```python
from build123d import *

# Parameters (mm, degrees)
F0_W          = 3
F0_H          = 80
F2_R          = 12.5
F3_DEPTH      = 119.80777
F4_R          = 15
F5_DEPTH      = 102.88035
F4_R_2        = 18
F6_DEPTH      = 2
F6_DEPTH_BACK = 28
F7_R          = 1.99999


# Not quite as in the source:
# - a fillet or chamfer is up to 0.001 mm smaller than in the source, because OpenCascade refuses the exact size


with BuildPart() as f1:
    # F0 (on Front) → F1 (revolve)
    with BuildSketch(Plane.XZ):
        with Locations((11.5, -40)):
            Rectangle(F0_W, F0_H)
        with BuildLine():
            Line((10, -80), (10, 0))
            Line((10, 0), (0, 0))
            Line((0, 0), (-10, 0))
            Line((-10, 0), (-10, -80))
            add(Edge.make_bspline(
                [(-10, -80), (-6, -75.3330111863), (0, -64.6669888505), (6, -75.3330111128), (10, -80)],
                knots=[0, 0, 0, 0, 0.5, 1, 1, 1, 1], degree=3))
        make_face()
        with Locations((-11.5, -40)):
            Rectangle(F0_W, F0_H)
    revolve(axis=Axis((-1.5, 0, 0), (-1, 0, 0)))

    # F2 (on face) → F3 (cut)
    with BuildSketch(Plane(origin=(-13, 0, 0), x_dir=(0, -1, 0), z_dir=(-1, 0, 0))):
        with Locations((-43.3012701892, 25)):
            Circle(F2_R)
        with Locations((43.3012701892, 25)):
            Circle(F2_R)
        with Locations((43.3012701892, -25)):
            Circle(F2_R)
        with Locations((0, -50)):
            Circle(F2_R)
        with Locations((-43.3012701892, -25)):
            Circle(F2_R)
        with Locations((0, 50)):
            Circle(F2_R)
    extrude(amount=-F3_DEPTH, mode=Mode.SUBTRACT)

    # F4 (on face) → F5 (cut)
    with BuildSketch(Plane(origin=(-13, 0, 0), x_dir=(0, -1, 0), z_dir=(-1, 0, 0))):
        Circle(F4_R)
    extrude(amount=-F5_DEPTH, mode=Mode.SUBTRACT)

    # F4 (on face) → F6 (join, two sides)
    with BuildSketch(Plane(origin=(-13, 0, 0), x_dir=(0, -1, 0), z_dir=(-1, 0, 0))) as f6_sk:
        Circle(F4_R_2)
        Circle(F4_R, mode=Mode.SUBTRACT)
    extrude(amount=F6_DEPTH)
    extrude(f6_sk.sketch, amount=-F6_DEPTH_BACK)

    # F7 (radius 2 in the source; OpenCascade refuses exactly that, so slightly less here)
    f7_edges = [f1.edges().sort_by_distance(p)[0] for p in [
        (-15, 18, 0),
        (15, 18, 0),
    ]]
    fillet(f7_edges, radius=F7_R)


solid = f1.part
```
Check sheet for the modelled part. Datum: model origin and axes. Units: mm. Round coordinates to 2 decimals unless told otherwise and drop trailing zeros. Write item = value, one per line. Start each with the question number.
1) Thickness scan on probe 1 along Z at (x, y) = (2.5, 0); probe 2 along Z at (x, y) = (4.5, 4.5); probe 3 along Y at (x, z) = (10.5, -20). Record the ranges inside material, lowest first.
2) Sectioned sample at A-A, the plane y = 0. State how many separate pieces and enclosed holes the cut face has, plus the area to 3 significant figures.
3) Gauge pin test, flat ends, axial feed: pin 1 Ø4 at (x, z) = (-9.5, 53.5) entering from +Y; pin 2 Ø12 at (x, z) = (4.5, -44.5) entering from -Y; pin 3 Ø6 at (x, y) = (4.5, 8) entering from -Z. Record the tip position at first contact, or that the pin passes through.
4) Release check for a two-part mould opening along Z. For faces 1 (the cylindrical face through (-11.48, 78.1, 17.34)), 2 (the cylindrical face through (-0.21, 14.985, 0.66)), 3 (the flat face through (-13, -19, 1)), 4 (the cylindrical face through (-0.182, -54.848, 20.212)) record: released by +Z, released by -Z, zero draft, split by the parting line, or undercut.
Results are:
q1.probe_1 = -71.09 to -62.5, -37.5 to -15, 15 to 37.5, 62.5 to 71.09
q1.probe_2 = -72.96 to -61.66, -38.34 to -14.31, 14.31 to 38.34, 61.66 to 72.96
q1.probe_3 = -77.46 to -54.76, -31.84 to 31.84, 54.76 to 77.46
q2.separate_pieces = 4
q2.enclosed_holes = 0
q2.area = 1,860 mm^2
q3.pin_1 = 61.17
q3.pin_2 = -68.03
q3.pin_3 = -76.49
q4.face_1 = split by the parting line
q4.face_2 = undercut
q4.face_3 = zero draft
q4.face_4 = undercut
